```python
from build123d import *

# Parameters (mm, degrees)
F0_W     = 31.75
F0_H     = 31.75
F0_W_2   = 26.67
F0_H_2   = 26.67
F1_DEPTH = 85.725
F3_DEPTH = 31.75


with BuildPart() as f1:
    # F0 (on Front) → F1 (new body, symmetric)
    with BuildSketch(Plane.XZ):
        Rectangle(F0_W, F0_H)
        Rectangle(F0_W_2, F0_H_2, mode=Mode.SUBTRACT)
    extrude(amount=F1_DEPTH, both=True)

    # F2 (on face) → F3 (cut, through all)
    with BuildSketch(Plane(origin=(0, 0, -15.875), x_dir=(1, 0, 0), z_dir=(0, 0, -1))):
        Polygon((0, -80.225739), (-3.175, -85.725), (3.175, -85.725), align=None)
    extrude(amount=-F3_DEPTH, mode=Mode.SUBTRACT)


solid = f1.part
```
Check sheet for the modelled part. Datum: model origin and axes. Units: mm. A direction names the side the tool comes from. Give positions to 0.01 mm unless a question says otherwise; leave off trailing zeros. Order: outer loops, then holes, each group sorted by start corner. A loop starts at its lowest first (then second) coordinate and runs counter-clockwise, first axis right, second up. Notation, with made-up numbers: M -14.5,30 L -7.5,30 A33 cw -7.5,60 Z; hole C 48.25,-2.75 d8. An arc over 180 degrees is marked long. Answer in a Markdown table with one row per item. Add a question column.
Q1. Thickness scan on L1, parallel to Z at x = 9.5, y = 36 (3 decimals); L2, parallel to Y at x = -2.5, z = 14 (3 decimals). Record the ranges inside material, lowest first.
Q2. Release check for a two-part mould opening along X. For faces 1 (the flat face through (14, 85.725, 0)), 2 (the flat face through (-15.875, -1, 0)), 3 (the flat face through (-1.565, 82.937, -14.623)) record: released by +X, released by -X, zero draft, split by the parting line, or undercut.
Q3. Access from +Z, -Z, +X, -X, +Y, -Y to the whole of each face (thin tool, end or side, straight path). Record for faces 4 (the flat face through (15.875, -1, 0)), 5 (the flat face through (0, -1, 13.335)), 6 (the flat face through (1.6, 83, -14.6)).
Q4. Sectioned sample at B-B, the plane x = -5.5. Record the boundary of the cut face in (y, z) (3 decimals), and give its area (3 significant figures).
Q5. Sectioned sample at A-A, the plane z = 8. Record the boundary of the cut face in (x, y) (3 decimals), and give its area (3 significant figures).
Q6. Sectioned sample at C-C, the plane y = 66. Record the boundary of the cut face in (x, z) (3 decimals).
Verdict:
| question | item | result |
|---|---|---|
| 1 | L1 | -15.875 to -13.335, 13.335 to 15.875 |
| 1 | L2 | -85.725 to 84.556 |
| 2 | face 1 | zero draft |
| 2 | face 2 | released by -X |
| 2 | face 3 | undercut |
| 3 | face 4 | +Z, -Z, +X, +Y, -Y |
| 3 | face 5 | +Y, -Y |
| 3 | face 6 | +Z, -Z, +Y |
| 4 | outline | M -85.725,-15.875 L 85.725,-15.875 L 85.725,-13.335 L -85.725,-13.335 Z; M -85.725,13.335 L 85.725,13.335 L 85.725,15.875 L -85.725,15.875 Z |
| 4 | area | 871 mm² |
| 5 | outline | M -15.875,-85.725 L -13.335,-85.725 L -13.335,85.725 L -15.875,85.725 Z; M 13.335,-85.725 L 15.875,-85.725 L 15.875,85.725 L 13.335,85.725 Z |
| 5 | area | 871 mm² |
| 6 | outline | M -15.875,-15.875 L 15.875,-15.875 L 15.875,15.875 L -15.875,15.875 Z; hole M -13.335,-13.335 L 13.335,-13.335 L 13.335,13.335 L -13.335,13.335 Z |
